Solid Edge part; units mm, degrees
sketch "Sketch1" plane through (0, 0, 0) normal (0, 0, 1) x (1, 0, 0)
  line L0 (-12.8, -1.3) -> (-12.8, -16.5)
  line L1 (-12.8, -16.5) -> (-13.8, -16.5)
  line L2 (-13.8, -16.5) -> (-13.8, -15)
  line L3 (-13.8, -15) -> (-16.8, -15)
  line L4 (-16.8, -15) -> (-16.8, 0)
  line L5 (-16.8, 0) -> (16.8, 0)
  line L6 (16.8, -15) -> (16.8, 0)
  line L7 (13.8, -15) -> (16.8, -15)
  line L8 (13.8, -16.5) -> (13.8, -15)
  line L9 (12.8, -16.5) -> (13.8, -16.5)
  line L10 (12.8, -1.3) -> (12.8, -16.5)
  line L11 (12.5, -1.3) -> (12.8, -1.3)
  line L12 (12.5, -1) -> (12.5, -1.3)
  line L13 (-12.5, -1) -> (12.5, -1)
  line L14 (-12.5, -1) -> (-12.5, -1.3)
  line L15 (-12.8, -1.3) -> (-12.5, -1.3)
revolve "RevolvedProtrusion1" add sketch "Sketch1" angle 360 about axis through (-16.5, 0, 0) along (1, 0, 0)
fillet "Round1" radius 0.3 4 edges at (-16.8, 0, 15) (-12.8, 0, 16.5) (12.8, 0, 16.5) (16.8, 0, 15)
chamfer "Chamfer_1" distance 0.3 angle 45 2 edges at (-13.8, 0, 16.5) (13.8, 0, 16.5)
sketch "Sketch2" plane through (-16.8, 0, 0) normal (-1, 0, 0) x (0, -1, 0)
  line L0 (-7.9783, 0.5885) -> (-4.4989, -6.6152)
  line L1 (-4.4989, -6.6152) -> (3.4795, -7.2037)
  line L2 (3.4795, -7.2037) -> (7.9783, -0.5885)
  line L3 (7.9783, -0.5885) -> (4.4989, 6.6152)
  line L4 (4.4989, 6.6152) -> (-3.4795, 7.2037)
  line L5 (-3.4795, 7.2037) -> (-7.9783, 0.5885)
extrude "ExtrudedCutout_1" cut sketch "Sketch2" against normal blind 1.5
sketch "Sketch3" plane through (16.8, 0, 0) normal (1, 0, 0) x (0, 1, 0)
  line L0 (-6.0918, 5.1855) -> (-7.5367, -2.6829)
  line L1 (-7.5367, -2.6829) -> (-1.4449, -7.8684)
  line L2 (-1.4449, -7.8684) -> (6.0918, -5.1855)
  line L3 (6.0918, -5.1855) -> (7.5367, 2.6829)
  line L4 (7.5367, 2.6829) -> (1.4449, 7.8684)
  line L5 (1.4449, 7.8684) -> (-6.0918, 5.1855)
extrude "ExtrudedCutout_2" cut sketch "Sketch3" against normal blind 1.5
Design review of the part built by this model. Coordinates are the model's own, in mm. A direction names the side the tool comes from. Coordinates: 2 decimals unless noted, no trailing zeros. Order: outer loops, then holes, each group sorted by start corner. A loop starts at its lowest first (then second) coordinate and runs counter-clockwise, first axis right, second up. Notation, with made-up numbers: (-22.75, -21.75) -> (0.25, -21.75) arc R32 ccw to (0.25, 12.25) -> close; hole circle Ø3 at (4, 49.25). An arc over 180 degrees is marked (long way). One line per item, written item: value.
1) We need section A-A, the plane x = 7. Give the boundary of the cut face in (y, z), then the cut area to 3 significant figures.
Output values:
outline: circle Ø2 at (0, 0)
area: 3.14 mm2
2) Clearance check with flat-ended pins moving along their axes: P1, Ø7.5, axis at y = -2, z = -3, coming from the +X side; P2, Ø3, axis at y = 0.5, z = 0, coming from the -X side; P3, Ø4, axis at x = 12.5, y = 13, coming from the +Z side; P4, Ø3, axis at x = -11.5, y = 2.5, coming from the +Z side. State where each tip first meets the part, or that it passes through.
Output values:
P1: stops at x = 16.8
P2: stops at x = -15.3
P3: stops at z = 12.22
P4: stops at z = 16.32
3) Draft analysis for pull direction X (two halves, no side actions). For faces 4 (the face through (16.8, -3, -7)), 5 (the face through (-16.061, 0.566, -6.905)), 6 (the face through (-12.65, 0.17, -1.29)), state which applies: +X half, -X half, draft (parallel to the pull), parting line (faces both ways), or undercut.
Output values:
face 4: +X half
face 5: draft
face 6: undercut
4) To check wall thickness, follow probe 1 along X at (y, z) = (-7, -14); probe 2 along X at (y, z) = (-9, 2); probe 3 along Z at (x, y) = (-12, 0). State the ranges of each line that lie inside material, in increasing order. Write a range as [from, to].
Output values:
probe 1: x = [-13.8, -12.8], [12.8, 13.8]
probe 2: x = [-16.8, -12.8], [12.8, 16.8]
probe 3: z = [-1, 1]
5) Machinability: for faces 1 (the face through (-16.061, -6.263, 2.963)), 2 (the face through (-13.3, -15.24, -6.32)), 3 (the face through (16.061, 2.271, -6.546)), which of the approach directions +Z, -Z, +X, -X, +Y, -Y give a long, thin tool a straight path to every point of the face, cutting with its end or side? Answer none if there is none.
Output values:
face 1: -X
face 2: +X, -X
face 3: +X
